```python
from build123d import *

# Parameters (mm, degrees)
SKETCH5_W               = 1.587499994
SKETCH5_H               = 55.780081988
SKETCH7_R               = 1.5875
CUT_EXTRUDE5_DEPTH      = 10.524999994
CUT_EXTRUDE5_DEPTH_BACK = 10.524999994
SKETCH6_R               = 1.5875
CUT_EXTRUDE6_DEPTH      = 10.525000094
CUT_EXTRUDE6_DEPTH_BACK = 10.525000094
CUT_EXTRUDE7_START      = 77.941582
SKETCH8_R               = 12.7
CUT_EXTRUDE7_DEPTH      = 22.225
SKETCH10_R              = 7.9375
BOSS_EXTRUDE1_DEPTH     = 30.380082


with BuildPart() as part:
    # Sketch5 → Revolve2 (revolve)
    with BuildSketch(Plane(origin=(0, 0, 0), x_dir=(1, 0, 0), z_dir=(0, 1, 0))):
        with Locations((8.731249997, -50.051540994)):
            Rectangle(SKETCH5_W, SKETCH5_H)
    revolve(axis=Axis((0, 0, 0), (0, 0, 1)))

    # Sketch7 → Cut-Extrude5 (cut, two sides)
    with BuildSketch(Plane(origin=(0, 0, 0), x_dir=(0, 0, -1), z_dir=(1, 0, 0))) as cut_extrude5_sk:
        with Locations((-39.195999993, 0)):
            Circle(SKETCH7_R)
    extrude(amount=CUT_EXTRUDE5_DEPTH, mode=Mode.SUBTRACT)
    extrude(cut_extrude5_sk.sketch, amount=-CUT_EXTRUDE5_DEPTH_BACK, mode=Mode.SUBTRACT)

    # Sketch6 → Cut-Extrude6 (cut, two sides)
    with BuildSketch(Plane(origin=(0, 0, 0), x_dir=(1, 0, 0), z_dir=(0, 1, 0))) as cut_extrude6_sk:
        with Locations((1e-09, -33.163499999)):
            Circle(SKETCH6_R)
    extrude(amount=CUT_EXTRUDE6_DEPTH, mode=Mode.SUBTRACT)
    extrude(cut_extrude6_sk.sketch, amount=-CUT_EXTRUDE6_DEPTH_BACK, mode=Mode.SUBTRACT)

    # Sketch8 → Cut-Extrude7 (cut)
    with BuildSketch(Plane.XY.offset(CUT_EXTRUDE7_START)):
        Circle(SKETCH8_R)
        Polygon((9.235721046, -0.808020891), (8.681700155, -0.254), (8.681700155, 0.254), (9.235721046, 0.808020891), (8.593912259, 1.257420242), (8.505698985, 1.75770258), (8.955098336, 2.399511367), (8.245002688, 2.730634406), (8.071256455, 3.207998257), (8.402379494, 3.918093905), (7.645572882, 4.120879625), (7.391572882, 4.56082053), (7.594358603, 5.317627141), (6.813836213, 5.385914002), (6.487300108, 5.775064579), (6.555586968, 6.555586968), (5.775064579, 6.487300108), (5.385914002, 6.813836213), (5.317627141, 7.594358603), (4.56082053, 7.391572882), (4.120879625, 7.645572882), (3.918093905, 8.402379494), (3.207998257, 8.071256455), (2.730634406, 8.245002688), (2.399511367, 8.955098336), (1.75770258, 8.505698985), (1.257420242, 8.593912259), (0.808020891, 9.235721046), (0.254, 8.681700155), (-0.254, 8.681700155), (-0.808020891, 9.235721046), (-1.257420242, 8.593912259), (-1.75770258, 8.505698985), (-2.399511367, 8.955098336), (-2.730634406, 8.245002688), (-3.207998257, 8.071256455), (-3.918093905, 8.402379494), (-4.120879625, 7.645572882), (-4.56082053, 7.391572882), (-5.317627141, 7.594358603), (-5.385914002, 6.813836213), (-5.775064579, 6.487300108), (-6.555586968, 6.555586968), (-6.487300108, 5.775064579), (-6.813836213, 5.385914002), (-7.594358603, 5.317627141), (-7.391572882, 4.56082053), (-7.645572882, 4.120879625), (-8.402379494, 3.918093905), (-8.071256455, 3.207998257), (-8.245002688, 2.730634406), (-8.955098336, 2.399511367), (-8.505698985, 1.75770258), (-8.593912259, 1.257420242), (-9.235721046, 0.808020891), (-8.681700155, 0.254), (-8.681700155, -0.254), (-9.235721046, -0.808020891), (-8.593912259, -1.257420242), (-8.505698985, -1.75770258), (-8.955098336, -2.399511367), (-8.245002688, -2.730634406), (-8.071256455, -3.207998257), (-8.402379494, -3.918093905), (-7.645572882, -4.120879625), (-7.391572882, -4.56082053), (-7.594358603, -5.317627141), (-6.813836213, -5.385914002), (-6.487300108, -5.775064579), (-6.555586968, -6.555586968), (-5.775064579, -6.487300108), (-5.385914002, -6.813836213), (-5.317627141, -7.594358603), (-4.56082053, -7.391572882), (-4.120879625, -7.645572882), (-3.918093905, -8.402379494), (-3.207998257, -8.071256455), (-2.730634406, -8.245002688), (-2.399511367, -8.955098336), (-1.75770258, -8.505698985), (-1.257420242, -8.593912259), (-0.808020891, -9.235721046), (-0.254, -8.681700155), (0.254, -8.681700155), (0.808020891, -9.235721046), (1.257420242, -8.593912259), (1.75770258, -8.505698985), (2.399511367, -8.955098336), (2.730634406, -8.245002688), (3.207998257, -8.071256455), (3.918093905, -8.402379494), (4.120879625, -7.645572882), (4.56082053, -7.391572882), (5.317627141, -7.594358603), (5.385914002, -6.813836213), (5.775064579, -6.487300108), (6.555586968, -6.555586968), (6.487300108, -5.775064579), (6.813836213, -5.385914002), (7.594358603, -5.317627141), (7.391572882, -4.56082053), (7.645572882, -4.120879625), (8.402379494, -3.918093905), (8.071256455, -3.207998257), (8.245002688, -2.730634406), (8.955098336, -2.399511367), (8.505698985, -1.75770258), (8.593912259, -1.257420242), align=None, mode=Mode.SUBTRACT)
    extrude(amount=-CUT_EXTRUDE7_DEPTH, mode=Mode.SUBTRACT)

    # Sketch10 → Boss-Extrude1 (add)
    with BuildSketch(Plane(origin=(0, 0, 47.5615), x_dir=(-1, 0, 0), z_dir=(0, 0, -1))):
        Circle(SKETCH10_R)
    extrude(amount=-BOSS_EXTRUDE1_DEPTH)


solid = part.part
```
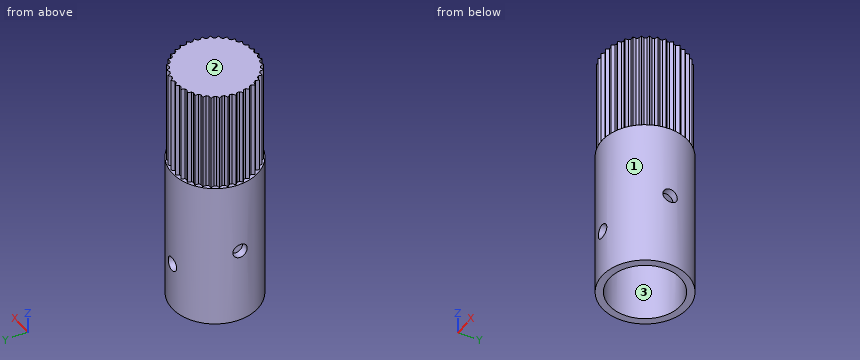
Part model, mm, in its own coordinate system. Face numbers are marked on the shaded views. Round coordinates to 2 decimals unless told otherwise and drop trailing zeros. Answer as CSV lines item,"result". Start each with the question number.
1) Drill centre lines: L1, parallel to Z at x = 9.05, y = 0; L2, parallel to Z at x = 0, y = 8.5; L3, parallel to Y at x = 0, z = 40 (1 decimal). Where is each one in solid material? Low to high.
2) Drop flat-ended pins along their axis: pin 1 (0.6 mm diameter, centred on x = 0, z = 67, fed in from -Y); pin 2 (5 mm diameter, centred on x = 3.5, y = -1, fed in from -Z); pin 3 (8 mm diameter, centred on x = 3.5, z = 34.5, fed in from +Y) (3 decimals); pin 4 (1.5 mm diameter, centred on y = -5.5, z = 54.5, fed in from +X). Give the stop position or say it passes through.
3) Mould opens along X. For the marked faces 1, 2 and 3 say: +X half, -X half, draft (parallel to the pull), parting line (faces both ways), or undercut.
Worked out:
1,L1,"22.16 to 37.61, 40.78 to 55.72"
1,L2,"22.16 to 31.58, 34.75 to 77.94"
1,L3,"-9.5 to -7.9, 7.9 to 9.5"
2,pin 1,"y = -8.73"
2,pin 2,"z = 47.56"
2,pin 3,"y = 9.525"
2,pin 4,"x = 8.26"
3,face 1,"parting line"
3,face 2,"draft"
3,face 3,"undercut"
